Design review of the part built by this model. Coordinates are the model's own, in mm. A direction names the side the tool comes from. Coordinates: 2 decimals unless noted, no trailing zeros. Write each loop counter-clockwise with the first axis right and the second up, starting at its lowest first coordinate (ties: lowest second). Pieces come first, ordered by that corner, then holes. Notation, with made-up numbers: (26.25, -37.5) -> (68.25, -37.5) arc R35 cw to (68.25, -4.5) -> close; hole circle Ø8 at (77, -29). An arc over 180 degrees is marked (long way). Return JSON: item names as keys, results as strings. Group by question number.
from build123d import *

# Parameters (mm, degrees)
SKETCH1_W           = 32.5
SKETCH1_H           = 32.5
SKETCH1_W_2         = 22.5
SKETCH1_H_2         = 22.5
BOSS_EXTRUDE1_DEPTH = 35
BOSS_EXTRUDE2_DEPTH = 6
SKETCH3_R           = 2
CUT_EXTRUDE1_DEPTH  = 51.518560945
SKETCH4_W           = 22.5
SKETCH4_H           = 5
CUT_EXTRUDE2_DEPTH  = 29
SKETCH6_W           = 58.5
SKETCH6_H           = 5
BOSS_EXTRUDE3_DEPTH = 20
SKETCH5_R           = 2
CUT_EXTRUDE3_DEPTH  = 65.426799548
SKETCH7_R           = 2
CUT_EXTRUDE4_DEPTH  = 65.426799548
CHAMFER1_SIZE       = 2


with BuildPart() as part:
    # Sketch1 → Boss-Extrude1 (new body)
    with BuildSketch(Plane.XY):
        Rectangle(SKETCH1_W, SKETCH1_H)
        Rectangle(SKETCH1_W_2, SKETCH1_H_2, mode=Mode.SUBTRACT)
    extrude(amount=BOSS_EXTRUDE1_DEPTH)

    # Sketch2 → Boss-Extrude2 (add)
    with BuildSketch(Plane(origin=(0, 0, 0), x_dir=(-1, 0, 0), z_dir=(0, 0, -1))):
        Polygon((-16.25, -16.25), (-29.25, -16.25), (-29.25, 29.25), (29.25, 29.25), (29.25, -16.25), (16.25, -16.25), (16.25, 16.25), (-16.25, 16.25), align=None)
    extrude(amount=-BOSS_EXTRUDE2_DEPTH)

    # Sketch3 → Cut-Extrude1 (cut, through all)
    with BuildSketch(Plane.XY.offset(6)):
        with Locations((-22.75, -1.25)):
            Circle(SKETCH3_R)
        with Locations((0, 20)):
            Circle(SKETCH3_R)
        with Locations((22.75, -1.25)):
            Circle(SKETCH3_R)
    extrude(amount=-CUT_EXTRUDE1_DEPTH, mode=Mode.SUBTRACT)

    # Sketch4 → Cut-Extrude2 (cut)
    with BuildSketch(Plane.XY.offset(35)):
        with Locations((0, 13.75)):
            Rectangle(SKETCH4_W, SKETCH4_H)
    extrude(amount=-CUT_EXTRUDE2_DEPTH, mode=Mode.SUBTRACT)

    # Sketch6 → Boss-Extrude3 (add)
    with BuildSketch(Plane(origin=(0, 0, 0), x_dir=(-1, 0, 0), z_dir=(0, 0, -1))):
        with Locations((0, -13.75)):
            Rectangle(SKETCH6_W, SKETCH6_H)
    extrude(amount=BOSS_EXTRUDE3_DEPTH)

    # Sketch5 → Cut-Extrude3 (cut, through all)
    with BuildSketch(Plane(origin=(16.25, 0, 0), x_dir=(0, 0, -1), z_dir=(1, 0, 0))):
        with Locations((-20.5, 0)):
            Circle(SKETCH5_R)
    extrude(amount=-CUT_EXTRUDE3_DEPTH, mode=Mode.SUBTRACT)

    # Sketch7 → Cut-Extrude4 (cut, through all)
    with BuildSketch(Plane.XZ.offset(16.25)):
        with Locations(Location((-20, -7, 0), (0, 0, 270))):
            Circle(SKETCH7_R)
        with Locations(Location((20, -7, 0), (0, 0, 270))):
            Circle(SKETCH7_R)
        with Locations(Location((0, 20.5, 0), (0, 0, 270))):
            Circle(SKETCH7_R)
    extrude(amount=-CUT_EXTRUDE4_DEPTH, mode=Mode.SUBTRACT)

    # Chamfer1
    chamfer1_edges = [part.edges().sort_by_distance(p)[0] for p in [
        (-20, -16.25, -5),
        (20, -16.25, -5),
        (0, -16.25, 22.5),
        (-24.75, -1.25, 6),
        (-2, 20, 6),
        (20.75, -1.25, 6),
        (-16.25, 0, 22.5),
        (16.25, 0, 22.5),
    ]]
    chamfer(chamfer1_edges, length=CHAMFER1_SIZE)


solid = part.part
Q1. For faces 4 (the flat face through (16.25, -4, 17)), 5 (the flat face through (0, 11.25, 3)), 6 (the flat face through (-11.25, 2, 17)), list the 3-axis set-ups (+Z, -Z, +X, -X, +Y, -Y) from which the entire face can be reached by the end or side of a thin tool; tool diameter is ignored.
Q2. We need section B-B on z = -7. Write out the cut boundary in (x, y).
Q3. Wall thickness on L1, parallel to X at y = -13, z = -7; L2, parallel to Y at x = 0, z = 1; L3, parallel to X at y = 2, z = 25: over which ranges is each line inside the solid? List them lowest first.
Q4. For P1, Ø6.5, axis at y = 0, z = 20.5, coming from the -X side; P2, Ø3, axis at y = -8, z = 11, coming from the +X side; P3, Ø5, axis at x = -20, z = -7, coming from the -Y side; P4, Ø5, axis at x = 17, y = -9, coming from the +Z side, all flat-tipped, find the tip position at first contact; note any pin that passes through.
Q5. We need section C-C on x = 0. Write out the cut boundary in (y, z).
Q6. The part is to be moulded in two halves that separate along Y. For faces 1 (the flat face through (14, 16.25, 20)), 2 (the cylindrical face through (12.8, -1.2, 22.1)), 3 (the flat face through (0, 12, 6)), say which applies: +Y half, -Y half, draft (parallel to the pull), parting line (faces both ways), or undercut.
Q7. We need section A-A on z = 20.5. Write out the cut boundary in (x, y).
Q8. We need section D-D on y = 10.5. Write out the cut boundary in (x, z), plus the area to 3 significant figures.
Findings below:
{
 "1": {"face 4": "+Z, +X, +Y, -Y", "face 5": "+Z, -Z", "face 6": "+Z"},
 "2": {"outline": "(-29.25, -16.25) -> (-24, -16.25) -> (-22, -14.25) -> (-22, -11.25) -> (-29.25, -11.25) -> close; (-18, -14.25) -> (-16, -16.25) -> (16, -16.25) -> (18, -14.25) -> (18, -11.25) -> (-18, -11.25) -> close; (22, -14.25) -> (24, -16.25) -> (29.25, -16.25) -> (29.25, -11.25) -> (22, -11.25) -> close"},
 "3": {"L1": "x = -29.25 to -22, -18 to 18, 22 to 29.25", "L2": "y = -16.25 to -11.25, 11.25 to 18, 22 to 29.25", "L3": "x = -16.25 to -11.25, 11.25 to 16.25"},
 "4": {"P1": "stops at x = -15.5", "P2": "stops at x = 16.25", "P3": "stops at y = -14.75", "P4": "stops at z = 35"},
 "5": {"outline": "(-16.25, -20) -> (-11.25, -20) -> (-11.25, 18.5) -> (-14.25, 18.5) -> (-16.25, 16.5) -> close; (-16.25, 24.5) -> (-14.25, 22.5) -> (-11.25, 22.5) -> (-11.25, 35) -> (-16.25, 35) -> close; (11.25, 0) -> (18, 0) -> (18, 4) -> (16, 6) -> (11.25, 6) -> close; (22, 0) -> (29.25, 0) -> (29.25, 6) -> (24, 6) -> (22, 4) -> close"},
 "6": {"face 1": "+Y half", "face 2": "undercut", "face 3": "draft"},
 "7": {"outline": "(-16.25, -16.25) -> (-4, -16.25) -> (-2, -14.25) -> (-2, -11.25) -> (-11.25, -11.25) -> (-11.25, -2) -> (-14.25, -2) -> (-16.25, -4) -> close; (-16.25, 4) -> (-14.25, 2) -> (-11.25, 2) -> (-11.25, 16.25) -> (-16.25, 16.25) -> close; (2, -14.25) -> (4, -16.25) -> (16.25, -16.25) -> (16.25, -4) -> (14.25, -2) -> (11.25, -2) -> (11.25, -11.25) -> (2, -11.25) -> close; (11.25, 2) -> (14.25, 2) -> (16.25, 4) -> (16.25, 16.25) -> (11.25, 16.25) -> close"},
 "8": {"outline": "(-29.25, 0) -> (-11.25, 0) -> (-11.25, 35) -> (-16.25, 35) -> (-16.25, 6) -> (-29.25, 6) -> close; (11.25, 0) -> (29.25, 0) -> (29.25, 6) -> (16.25, 6) -> (16.25, 35) -> (11.25, 35) -> close", "area": "506 mm^2"}
}
